For this review, use the dimensioned drawing (mm, ordinates from the lowest corner) and the shaded views. Coordinates: 2 decimals unless noted, no trailing zeros. Loops run counter-clockwise (first coordinate to the right, second up) from the corner with the lowest first, then second, coordinate; pieces in that order, holes last. Notation, with made-up numbers: (80, 67) - (98, 67) arc R28 ccw to (98, 98) - close; hole circle Ø5 at (-28, 47). An arc over 180 degrees is marked (long way). Use a Markdown table: item, result. Add a question column.
1) Add section D-D, the plane x = 18. Give the boundary of the cut face in (y, z).
2) To check wall thickness, follow L1, parallel to Z at x = 10, y = 7.75; L2, parallel to X at y = 9.25, z = 4.75; L3, parallel to Z at x = 8.5, y = 2.75. State the ranges of each line that lie inside material, in increasing order. Write a range as [from, to].
3) Add section B-B, the plane z = 5. Give the boundary of the cut face in (x, y), and give its area (3 significant figures).
4) The part is to be moulded in two halves that separate along Y. For the marked faces 1, 2, 3 and 4, say which applies: pulls with the +Y half, pulls with the -Y half, needs draft (parallel to the pull), parting line crosses it, or undercut.
5) Clearance check with flat-ended pins moving along their axes: pin 1 (1 mm diameter, centred on x = 7.5, z = 1.5, fed in from -Y); pin 2 (1.5 mm diameter, centred on x = 11, y = 3, fed in from +Z); pin 3 (2 mm diameter, centred on x = 10, z = 5, fed in from +Y); pin 4 (2 mm diameter, centred on x = 6, z = 7, fed in from +Y). State where each tip first meets the part, or that it passes through.
6) Add section C-C, the plane x = 10. Give the boundary of the cut face in (y, z), and give its area (3 significant figures).
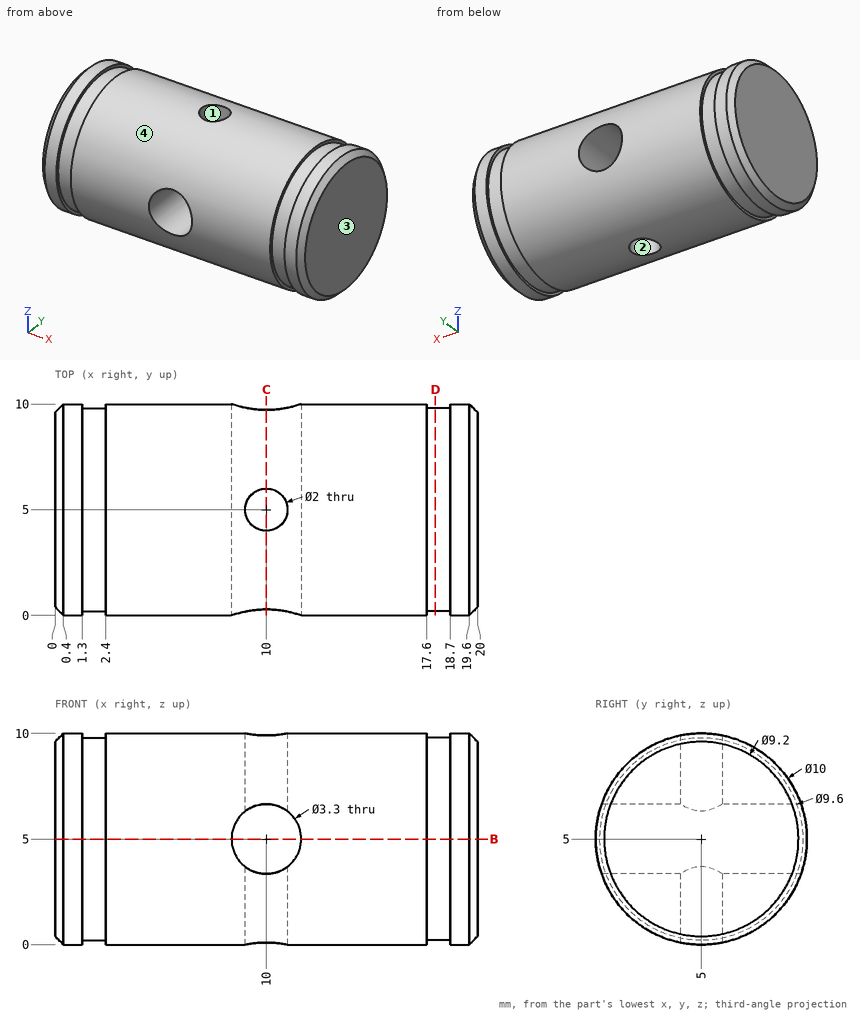
From the geometry:
| question | item | result |
|---|---|---|
| 1 | outline | circle Ø9.6 at (5, 5) |
| 2 | L1 | z = [0.82, 3.35], [6.65, 9.18] |
| 2 | L2 | x = [0, 8.37], [11.63, 20] |
| 2 | L3 | z = [0.53, 4.31], [5.69, 9.47] |
| 3 | outline | (0, 0.4) - (0.4, 0) - (1.3, 0) - (1.3, 0.2) - (2.4, 0.2) - (2.4, 0) - (8.35, 0) - (8.35, 10) - (2.4, 10) - (2.4, 9.8) - (1.3, 9.8) - (1.3, 10) - (0.4, 10) - (0, 9.6) - close; (11.65, 0) - (17.6, 0) - (17.6, 0.2) - (18.7, 0.2) - (18.7, 0) - (19.6, 0) - (20, 0.4) - (20, 9.6) - (19.6, 10) - (18.7, 10) - (18.7, 9.8) - (17.6, 9.8) - (17.6, 10) - (11.65, 10) - close |
| 3 | area | 166 mm^2 |
| 4 | face 1 | undercut |
| 4 | face 2 | undercut |
| 4 | face 3 | needs draft |
| 4 | face 4 | parting line crosses it |
| 5 | pin 1 | stops at y = 1 |
| 5 | pin 2 | stops at z = 9.84 |
| 5 | pin 3 | passes through |
| 5 | pin 4 | stops at y = 9.9 |
| 6 | outline | (0.28, 3.35) arc R5 ccw to (4, 0.1) - (4, 3.35) - close; (0.28, 6.65) - (4, 6.65) - (4, 9.9) arc R5 ccw to start; (6, 0.1) arc R5 ccw to (9.72, 3.35) - (6, 3.35) - close; (6, 6.65) - (9.72, 6.65) arc R5 ccw to (6, 9.9) - close |
| 6 | area | 32.9 mm^2 |
